from build123d import *

# Parameters (mm, degrees)
CROQUIS1_W              = 40
CROQUIS1_H              = 50
SALIENTE_EXTRUIR1_DEPTH = 5
CROQUIS2_R              = 1.25
CROQUIS2_R_2            = 2.25
CORTAR_EXTRUIR2_DEPTH   = 5
CROQUIS4_W              = 40
CROQUIS4_H              = 75
SALIENTE_EXTRUIR2_DEPTH = 5
REDONDEO1_R             = 7


with BuildPart() as part:
    # Croquis1 → Saliente-Extruir1 (new body)
    with BuildSketch(Plane.XY):
        with Locations((4.439140811, -9.15274463)):
            Rectangle(CROQUIS1_W, CROQUIS1_H)
    extrude(amount=SALIENTE_EXTRUIR1_DEPTH)

    # Croquis2 → Cortar-Extruir2 (cut)
    with BuildSketch(Plane.XY.offset(5)):
        with Locations((4.439140811, 0.84725537)):
            Circle(CROQUIS2_R)
        with Locations((4.439140811, -21.65274463)):
            Circle(CROQUIS2_R_2)
    extrude(amount=-CORTAR_EXTRUIR2_DEPTH, mode=Mode.SUBTRACT)

    # Croquis4 → Saliente-Extruir2 (add)
    with BuildSketch(Plane.XZ.offset(34.15274463)):
        with Locations((4.439140811, -32.5)):
            Rectangle(CROQUIS4_W, CROQUIS4_H)
    extrude(amount=SALIENTE_EXTRUIR2_DEPTH)

    # Redondeo1
    redondeo1_edges = [part.edges().sort_by_distance(p)[0] for p in [
        (4.439140811, -39.15274463, 5),
    ]]
    fillet(redondeo1_edges, radius=REDONDEO1_R)


solid = part.part
Verification items for the finished model (mm, model axes). A direction names the side the tool comes from. Round coordinates to 2 decimals unless told otherwise and drop trailing zeros. Loops run counter-clockwise (first coordinate to the right, second up) from the corner with the lowest first, then second, coordinate; pieces in that order, holes last. Notation, with made-up numbers: (33, 67) - (46, 67) arc R4 ccw to (46, 74) - close; hole circle Ø5 at (38, -39.75). An arc over 180 degrees is marked (long way). Use a Markdown table: item, result. Add a question column.
1. Access from +Z, -Z, +X, -X, +Y, -Y to the whole of each face (thin tool, end or side, straight path). Record for faces 1 (the face through (4.72, -37.05, 3)), 2 (the face through (4, -34.153, -35)).
2. Section check B-B, the plane y = 9. Record the boundary of the cut face in (x, z).
3. Gauge pin test, flat ends, axial feed: pin 1 (6 mm diameter, centred on x = 8.5, z = -27, fed in from +Y); pin 2 (8 mm diameter, centred on x = -6, y = -28.5, fed in from -Z). Record the tip position at first contact, or that the pin passes through.
4. Section check C-C, the plane z = -21. Record the boundary of the cut face in (x, y), plus the area to 3 significant figures.
5. Thickness scan on probe 1 along Y at (x, z) = (7.5, -33); probe 2 along Z at (x, y) = (10.5, 14.5). Record the ranges inside material, lowest first. Write a range as [from, to].
6. Section check A-A, the plane x = -5. Record the boundary of the cut face in (y, z).
7. Release check for a two-part mould opening along X. For faces 3 (the face through (24.439, -36, -19)), 4 (the face through (4, -39.153, -36)), 5 (the face through (4.15, -19.42, 2.54)) record: released by +X, released by -X, zero draft, split by the parting line, or undercut.
Checks:
| question | item | result |
|---|---|---|
| 1 | face 1 | +Z, +X, -X, -Y |
| 1 | face 2 | -Z, +X, -X, +Y |
| 2 | outline | (-15.56, 0) - (24.44, 0) - (24.44, 5) - (-15.56, 5) - close |
| 3 | pin 1 | stops at y = -34.15 |
| 3 | pin 2 | stops at z = 0 |
| 4 | outline | (-15.56, -39.15) - (24.44, -39.15) - (24.44, -34.15) - (-15.56, -34.15) - close |
| 4 | area | 200 mm^2 |
| 5 | probe 1 | y = [-39.15, -34.15] |
| 5 | probe 2 | z = [0, 5] |
| 6 | outline | (-39.15, -70) - (-34.15, -70) - (-34.15, 0) - (15.85, 0) - (15.85, 5) - (-32.15, 5) arc R7 ccw to (-39.15, -2) - close |
| 7 | face 3 | released by +X |
| 7 | face 4 | zero draft |
| 7 | face 5 | undercut |
